The drawing under review shows one solid part. Ordinate dimensions are in mm from its lowest x, y, z. A direction names the side the tool comes from. Give positions to 0.01 mm unless a question says otherwise; leave off trailing zeros. Write each loop counter-clockwise with the first axis right and the second up, starting at its lowest first coordinate (ties: lowest second). Pieces come first, ordered by that corner, then holes. Notation, with made-up numbers: (-8.75, 47.5) - (21.25, 47.5) arc R13 cw to (21.25, 69.5) - close; hole circle Ø1 at (74.25, 0.25). An arc over 180 degrees is marked (long way). Write each question's results on one line, items separated by ' | '. Start each with the question number.
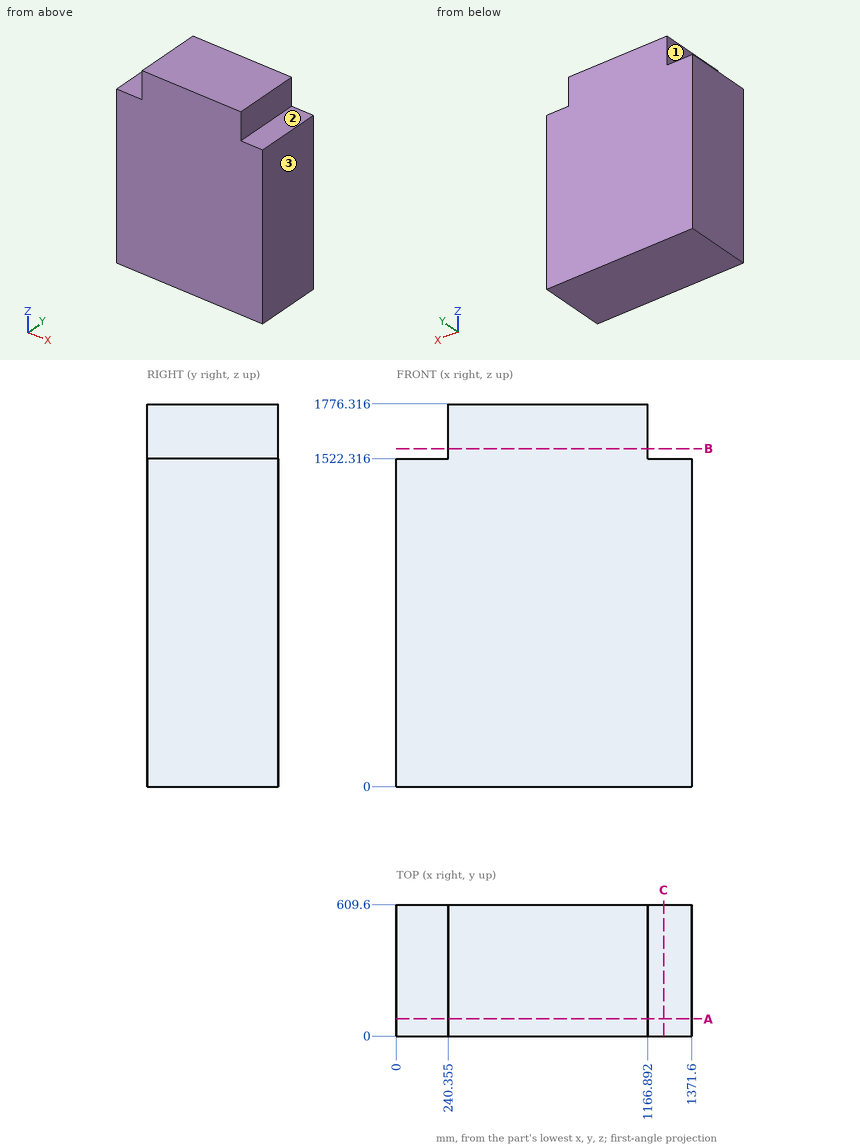
Q1. Add section A-A on y = 79.5. State the section outline as (x, z) points (1 decimal), plus the area to 3 significant figures.
Q2. For line 1 along Z through (x, y) = (1293.5, 36) (1 decimal); line 2 along X through (y, z) = (427.5, 1650) (1 decimal), list the stretches that pass through material, from the lowest coordinate up. Write a range as [from, to].
Q3. Machinability: for the marked faces 1, 2 and 3, which of the approach directions +Z, -Z, +X, -X, +Y, -Y give a long, thin tool a straight path to every point of the face, cutting with its end or side? Answer none if there is none.
Q4. Add section C-C on x = 1240. State the section outline as (y, z) points (1 decimal), plus the area to 3 significant figures.
Q5. Add section B-B on z = 1569. State the section outline as (x, y) points (1 decimal).
Q6. Insertion check: P1, Ø10, axis at x = 960, z = 1029.5, coming from the -Y side; P2, Ø1.5, axis at x = 193.5, y = 285, coming from the +Z side. Each pin has a flat end and moves straight along its axis. Give the tip position at first contact, or say it passes through.
Result:
1) outline: (0, 0) - (1371.6, 0) - (1371.6, 1522.3) - (1166.9, 1522.3) - (1166.9, 1776.3) - (240.4, 1776.3) - (240.4, 1522.3) - (0, 1522.3) - close | area: 2,320,000 mm²
2) line 1: z = [0, 1522.3] | line 2: x = [240.4, 1166.9]
3) face 1: +Z, -X, +Y, -Y | face 2: +Z, +X, +Y, -Y | face 3: +Z, -Z, +X, +Y, -Y
4) outline: (0, 0) - (609.6, 0) - (609.6, 1522.3) - (0, 1522.3) - close | area: 928,000 mm²
5) outline: (240.4, 0) - (1166.9, 0) - (1166.9, 609.6) - (240.4, 609.6) - close
6) P1: stops at y = 0 | P2: stops at z = 1522.32
